Model file for the job. Use its own axes, mm. A direction names the side the tool comes from. Round coordinates to 2 decimals unless told otherwise and drop trailing zeros. Write each loop counter-clockwise with the first axis right and the second up, starting at its lowest first coordinate (ties: lowest second). Pieces come first, ordered by that corner, then holes. Notation, with made-up numbers: (72.5, -39.75) - (88.5, -39.75) arc R29 cw to (88.5, -4.75) - close; hole circle Ø2 at (69, 48). An arc over 180 degrees is marked (long way). One line per item, written item: value.
from build123d import *

# Parameters (mm, degrees)
SKETCH1_R           = 0.889
SKETCH1_R_2         = 1.85293
SKETCH1_W           = 12.25
SKETCH1_H           = 24
BOSS_EXTRUDE1_DEPTH = 6.35


with BuildPart() as part:
    # Sketch1 → Boss-Extrude1 (new body)
    with BuildSketch(Plane(origin=(0, 0, 0), x_dir=(1, 0, 0), z_dir=(0, 1, 0))):
        with BuildLine():
            Line((-25.79604899, 10.914446368), (-25.79604899, 28.914446368))
            Line((-25.79604899, 28.914446368), (-25.79604899, 30.914446368))
            ThreePointArc((-25.79604899, 30.914446368), (-25.503155771, 31.621553149), (-24.79604899, 31.914446368))
            Line((-24.79604899, 31.914446368), (-22.169032336, 31.914446368))
            ThreePointArc((-22.169032336, 31.914446368), (-21.5566599, 31.705015783), (-21.200786499, 31.164446368))
            ThreePointArc((-21.200786499, 31.164446368), (-17.918036112, 28.938357279), (-15.29604899, 31.914446368))
            Line((-15.29604899, 31.914446368), (-15.29604899, 34.914446368))
            ThreePointArc((-15.29604899, 34.914446368), (-17.918036112, 37.890535457), (-21.200786499, 35.664446368))
            ThreePointArc((-21.200786499, 35.664446368), (-21.5566599, 35.123876953), (-22.169032336, 34.914446368))
            Line((-22.169032336, 34.914446368), (-24.718665279, 34.914446368))
            ThreePointArc((-24.718665279, 34.914446368), (-25.478219804, 35.264002732), (-25.706760093, 36.068292522))
            ThreePointArc((-25.706760093, 36.068292522), (-17.717401115, 42.392090826), (-10.79604899, 34.914446368))
            Line((-10.79604899, 34.914446368), (-10.79604899, 34.414446368))
            ThreePointArc((-10.79604899, 34.414446368), (-9.185136286, 30.525359071), (-5.29604899, 28.914446368))
            Line((-5.29604899, 28.914446368), (18.70395101, 28.914446368))
            ThreePointArc((18.70395101, 28.914446368), (22.593038307, 30.525359071), (24.20395101, 34.414446368))
            Line((24.20395101, 34.414446368), (24.20395101, 34.914446368))
            ThreePointArc((24.20395101, 34.914446368), (31.125303135, 42.392090826), (39.114662113, 36.068292522))
            ThreePointArc((39.114662113, 36.068292522), (38.886121825, 35.264002732), (38.126567299, 34.914446368))
            Line((38.126567299, 34.914446368), (35.576934356, 34.914446368))
            ThreePointArc((35.576934356, 34.914446368), (34.964561921, 35.123876953), (34.60868852, 35.664446368))
            ThreePointArc((34.60868852, 35.664446368), (31.325938133, 37.890535457), (28.70395101, 34.914446368))
            Line((28.70395101, 34.914446368), (28.70395101, 31.914446368))
            ThreePointArc((28.70395101, 31.914446368), (31.325938133, 28.938357279), (34.60868852, 31.164446368))
            ThreePointArc((34.60868852, 31.164446368), (34.964561921, 31.705015783), (35.576934356, 31.914446368))
            Line((35.576934356, 31.914446368), (38.20395101, 31.914446368))
            ThreePointArc((38.20395101, 31.914446368), (38.911057791, 31.621553149), (39.20395101, 30.914446368))
            Line((39.20395101, 30.914446368), (39.20395101, 28.914446368))
            Line((39.20395101, 28.914446368), (39.20395101, 10.914446368))
            ThreePointArc((39.20395101, 10.914446368), (31.88162054, -6.763223162), (14.20395101, -14.085553632))
            Line((14.20395101, -14.085553632), (-0.79604899, -14.085553632))
            ThreePointArc((-0.79604899, -14.085553632), (-18.47371852, -6.763223162), (-25.79604899, 10.914446368))
        make_face()
        with Locations((6.70395101, 19.714446368)):
            Circle(SKETCH1_R, mode=Mode.SUBTRACT)
        with Locations((6.70395101, -9.885553632)):
            Circle(SKETCH1_R, mode=Mode.SUBTRACT)
        with Locations((-18.29604899, 4.914446368)):
            Circle(SKETCH1_R_2, mode=Mode.SUBTRACT)
        with Locations((31.70395101, 4.914446368)):
            Circle(SKETCH1_R_2, mode=Mode.SUBTRACT)
        with Locations((6.70395101, 4.914446368)):
            Rectangle(SKETCH1_W, SKETCH1_H, mode=Mode.SUBTRACT)
        with BuildLine():
            Line((-9.42104899, 6.414446368), (-4.42104899, 6.414446368))
            ThreePointArc((-4.42104899, 6.414446368), (-2.92104899, 4.914446368), (-4.42104899, 3.414446368))
            Line((-4.42104899, 3.414446368), (-9.42104899, 3.414446368))
            ThreePointArc((-9.42104899, 3.414446368), (-10.92104899, 4.914446368), (-9.42104899, 6.414446368))
        make_face(mode=Mode.SUBTRACT)
        with BuildLine():
            Line((22.82895101, 3.414446368), (17.82895101, 3.414446368))
            ThreePointArc((17.82895101, 3.414446368), (16.32895101, 4.914446368), (17.82895101, 6.414446368))
            Line((17.82895101, 6.414446368), (22.82895101, 6.414446368))
            ThreePointArc((22.82895101, 6.414446368), (24.32895101, 4.914446368), (22.82895101, 3.414446368))
        make_face(mode=Mode.SUBTRACT)
        with BuildLine():
            Line((-9.42104899, -3.585553632), (-4.42104899, -3.585553632))
            ThreePointArc((-4.42104899, -3.585553632), (-2.92104899, -5.085553632), (-4.42104899, -6.585553632))
            Line((-4.42104899, -6.585553632), (-9.42104899, -6.585553632))
            ThreePointArc((-9.42104899, -6.585553632), (-10.92104899, -5.085553632), (-9.42104899, -3.585553632))
        make_face(mode=Mode.SUBTRACT)
        with BuildLine():
            Line((22.82895101, -6.585553632), (17.82895101, -6.585553632))
            ThreePointArc((17.82895101, -6.585553632), (16.32895101, -5.085553632), (17.82895101, -3.585553632))
            Line((17.82895101, -3.585553632), (22.82895101, -3.585553632))
            ThreePointArc((22.82895101, -3.585553632), (24.32895101, -5.085553632), (22.82895101, -6.585553632))
        make_face(mode=Mode.SUBTRACT)
        with BuildLine():
            Line((-9.42104899, 16.414446368), (-4.42104899, 16.414446368))
            ThreePointArc((-4.42104899, 16.414446368), (-2.92104899, 14.914446368), (-4.42104899, 13.414446368))
            Line((-4.42104899, 13.414446368), (-9.42104899, 13.414446368))
            ThreePointArc((-9.42104899, 13.414446368), (-10.92104899, 14.914446368), (-9.42104899, 16.414446368))
        make_face(mode=Mode.SUBTRACT)
        with BuildLine():
            Line((22.82895101, 13.414446368), (17.82895101, 13.414446368))
            ThreePointArc((17.82895101, 13.414446368), (16.32895101, 14.914446368), (17.82895101, 16.414446368))
            Line((17.82895101, 16.414446368), (22.82895101, 16.414446368))
            ThreePointArc((22.82895101, 16.414446368), (24.32895101, 14.914446368), (22.82895101, 13.414446368))
        make_face(mode=Mode.SUBTRACT)
        with BuildLine():
            Line((-9.42104899, 26.414446368), (-4.42104899, 26.414446368))
            ThreePointArc((-4.42104899, 26.414446368), (-2.92104899, 24.914446368), (-4.42104899, 23.414446368))
            Line((-4.42104899, 23.414446368), (-9.42104899, 23.414446368))
            ThreePointArc((-9.42104899, 23.414446368), (-10.92104899, 24.914446368), (-9.42104899, 26.414446368))
        make_face(mode=Mode.SUBTRACT)
        with BuildLine():
            Line((22.82895101, 23.414446368), (17.82895101, 23.414446368))
            ThreePointArc((17.82895101, 23.414446368), (16.32895101, 24.914446368), (17.82895101, 26.414446368))
            Line((17.82895101, 26.414446368), (22.82895101, 26.414446368))
            ThreePointArc((22.82895101, 26.414446368), (24.32895101, 24.914446368), (22.82895101, 23.414446368))
        make_face(mode=Mode.SUBTRACT)
    extrude(amount=BOSS_EXTRUDE1_DEPTH)


solid = part.part
1. Mould opens along X. For faces 1 (the face through (7, 3, 14.086)), 2 (the face through (22.55, 3.13, -30.48)), 3 (the face through (0.579, 3, -5)), 4 (the face through (39.204, 3, -21)) say: released by +X, released by -X, zero draft, split by the parting line, or undercut.
Report:
face 1: zero draft
face 2: undercut
face 3: undercut
face 4: released by +X
2. Drop flat-ended pins along their axis: pin 1 (2 mm diameter, centred on x = -24, y = 3.5, fed in from +Z); pin 2 (3 mm diameter, centred on y = 1.5, z = -2, fed in from +X); pin 3 (2.5 mm diameter, centred on x = -7.5, y = 2.5, fed in from +Z). Give the stop position or say it passes through.
Report:
pin 1: z = 0.57
pin 2: x = 38.08
pin 3: z = 13.48
3. Band-saw the part on B-B on x = -7. Write the cut outline in (y, z), plus the area to 3 significant figures.
Report:
outline: (0, -29.19) - (6.35, -29.19) - (6.35, -26.41) - (0, -26.41) - close; (0, -23.41) - (6.35, -23.41) - (6.35, -16.41) - (0, -16.41) - close; (0, -13.41) - (6.35, -13.41) - (6.35, -6.41) - (0, -6.41) - close; (0, -3.41) - (6.35, -3.41) - (6.35, 3.59) - (0, 3.59) - close; (0, 6.59) - (6.35, 6.59) - (6.35, 13.3) - (0, 13.3) - close
area: 194 mm²
4. Tool access for faces 5 (the face through (0, 6.35, -15)), 6 (the face through (16.33, 3.13, -24.88)), 7 (the face through (37, 3, -34.914)): list every direction of +Z, -Z, +X, -X, +Y, -Y with a clear straight run to the whole face (end or side of a thin tool).
Report:
face 5: +Z, -Z, +X, -X, +Y
face 6: +Y, -Y
face 7: +X, +Y, -Y
5. Wall check: probe 1 along Z at (x, y) = (19, 5.25); probe 2 along Z at (x, y) = (16.5, 5.5); probe 3 along X at (y, z) = (3.75, -6). Give the ranges that are in metal, low to high. Write a range as [from, to].
Report:
probe 1: [-28.92, -26.41], [-23.41, -16.41], [-13.41, -6.41], [-3.41, 3.59], [6.59, 13.62]
probe 2: [-28.91, -25.61], [-24.22, -15.61], [-14.22, -5.61], [-4.22, 4.39], [5.78, 13.98]
probe 3: [-25.31, -19.8], [-16.79, -10.46], [-3.39, 0.58], [12.83, 16.79], [23.86, 30.2], [33.21, 38.72]
6. Band-saw the part on A-A on z = -12. Write the cut outline in (x, y).
Report:
outline: (-25.8, 0) - (0.58, 0) - (0.58, 6.35) - (-25.8, 6.35) - close; (12.83, 0) - (39.2, 0) - (39.2, 6.35) - (12.83, 6.35) - close
7. Band-saw the part on C-C on x = -18.5. Write the cut outline in (y, z).
Report:
outline: (0, -42.41) - (6.35, -42.41) - (6.35, -37.91) - (0, -37.91) - close; (0, -28.92) - (6.35, -28.92) - (6.35, -6.76) - (0, -6.76) - close; (0, -3.07) - (6.35, -3.07) - (6.35, 6.74) - (0, 6.74) - close
8. Band-saw the part on D-D on z = -25. Write the cut outline in (x, y).
Report:
outline: (-25.8, 0) - (-10.92, 0) - (-10.92, 6.35) - (-25.8, 6.35) - close; (-2.92, 0) - (16.33, 0) - (16.33, 6.35) - (-2.92, 6.35) - close; (24.33, 0) - (39.2, 0) - (39.2, 6.35) - (24.33, 6.35) - close
